Geometry: final body of the model. Coordinates: model frame, mm. A direction names the side the tool comes from. Give positions to 0.01 mm unless a question says otherwise; leave off trailing zeros. Loops run counter-clockwise (first coordinate to the right, second up) from the corner with the lowest first, then second, coordinate; pieces in that order, holes last. Notation, with made-up numbers: (69.25, 88.25) - (94.25, 88.25) arc R19 ccw to (94.25, 103.25) - close; hole circle Ø11 at (56.25, 77.25). An arc over 180 degrees is marked (long way). Use one line per item in the form item = value.
```python
from build123d import *

# Parameters (mm, degrees)
SKETCH1_R           = 2.1
BOSS_EXTRUDE2_DEPTH = 3
SKETCH1_14_R        = 5
CUT_EXTRUDE2_DEPTH  = 10


with BuildPart() as part:
    # Sketch1 → Boss-Extrude2 (new body)
    with BuildSketch(Plane(origin=(0, 0, 0), x_dir=(1, 0, 0), z_dir=(0, 1, 0))):
        with BuildLine():
            Line((32, -25), (32, -14.320549047))
            Line((32, -14.320549047), (28.692414075, -11.736497543))
            ThreePointArc((28.692414075, -11.736497543), (31, 0), (28.692414075, 11.736497543))
            Line((28.692414075, 11.736497543), (32, 14.320549047))
            Line((32, 14.320549047), (32, 25))
            Line((32, 25), (-32, 25))
            Line((-32, 25), (-32, 14.320549047))
            Line((-32, 14.320549047), (-28.692414075, 11.736497543))
            ThreePointArc((-28.692414075, 11.736497543), (-31, 0), (-28.692414075, -11.736497543))
            Line((-28.692414075, -11.736497543), (-32, -14.320549047))
            Line((-32, -14.320549047), (-32, -25))
            Line((-32, -25), (32, -25))
        make_face()
        with Locations(Location((26, 0, 0), (0, 0, 270))):
            Circle(SKETCH1_R, mode=Mode.SUBTRACT)
        with Locations(Location((-26, 0, 0), (0, 0, 270))):
            Circle(SKETCH1_R, mode=Mode.SUBTRACT)
    extrude(amount=BOSS_EXTRUDE2_DEPTH)

    # Sketch1_14 → Cut-Extrude2 (cut)
    with BuildSketch(Plane(origin=(0, 0, 0), x_dir=(1, 0, 0), z_dir=(0, 1, 0))):
        with Locations(Location((0, 0, 0), (0, 0, 270))):
            Circle(SKETCH1_14_R)
    extrude(amount=CUT_EXTRUDE2_DEPTH, mode=Mode.SUBTRACT)


solid = part.part
```
(1) Access query for faces 5 (the face through (0, 1, 25)), 6 (the face through (-30.32, 1.48, 13.01)), 7 (the face through (30.32, 1.48, -13.01)). Directions: +Z, -Z, +X, -X, +Y, -Y. A direction counts if a zero-diameter tool reaches every point of the face in a straight line with its end or side. Return the directions, or none.
Solution:
face_5 = +Z, +X, -X, +Y, -Y
face_6 = -X, +Y, -Y
face_7 = +X, +Y, -Y
(2) Cut plane A-A (x = -26). Return the cut outline in (y, z), plus the area to 3 significant figures.
Solution:
outline = (0, -25) - (3, -25) - (3, -2.1) - (0, -2.1) - close; (0, 2.1) - (3, 2.1) - (3, 25) - (0, 25) - close
area = 137 mm2
(3) Cut plane C-C (z = 0). Return the cut outline in (x, y), plus the area to 3 significant figures.
Solution:
outline = (-31, 0) - (-28.1, 0) - (-28.1, 3) - (-31, 3) - close; (-23.9, 0) - (-5, 0) - (-5, 3) - (-23.9, 3) - close; (5, 0) - (23.9, 0) - (23.9, 3) - (5, 3) - close; (28.1, 0) - (31, 0) - (31, 3) - (28.1, 3) - close
area = 131 mm2
(4) Cut plane B-B (y = 2.45). Return the cut outline in (x, z), plus the area to 3 significant figures.
Solution:
outline = (-32, -25) - (32, -25) - (32, -14.32) - (28.69, -11.74) arc R31 ccw to (28.69, 11.74) - (32, 14.32) - (32, 25) - (-32, 25) - (-32, 14.32) - (-28.69, 11.74) arc R31 ccw to (-28.69, -11.74) - (-32, -14.32) - close; hole circle Ø4.2 at (-26, 0); hole circle Ø10 at (0, 0); hole circle Ø4.2 at (26, 0)
area = 2,990 mm2
(5) Pull-direction query (Z, two-part tool) for faces 1 (the face through (-4.88, 1.48, -1.08)), 2 (the face through (32, 1, -20)), 3 (the face through (-30.369, 1.479, -13.047)), 4 (the face through (0, 1, -25)); classes: released by +Z, released by -Z, zero draft, split by the parting line, or undercut.
Solution:
face_1 = undercut
face_2 = zero draft
face_3 = undercut
face_4 = released by -Z
(6) Cut plane D-D (x = 0). Return the cut outline in (y, z).
Solution:
outline = (0, -25) - (3, -25) - (3, -5) - (0, -5) - close; (0, 5) - (3, 5) - (3, 25) - (0, 25) - close
(7) Material intervals for L1, parallel to Z at x = 0, y = 2; L2, parallel to X at y = 1.6, z = 4.5; L3, parallel to Z at x = 26.5, y = 1.9, sorted ascending. Write a range as from..to.
Solution:
L1 = -25..-5, 5..25
L2 = -30.67..-2.18, 2.18..30.67
L3 = -25..-2.04, 2.04..25
